Source: CAD feature listing. Evaluate the final solid. Frame: model axes, mm. Give positions to 0.01 mm unless a question says otherwise; leave off trailing zeros. Use one line per item in the form item = value. Start each with the question number.
(1) Cut plane A-A, the plane z = 1.5. Count the separate pieces of the cut face and the enclosed holes in it, and give its area (3 significant figures).
(2) Material intervals for line 1 along X through (y, z) = (-18, 1.85); line 2 along X through (y, z) = (-4.5, 5); line 3 along Y through (x, z) = (-198.5, 1.2), sorted ascending. Write a range as from..to.
(3) First-contact query: P1, Ø3, axis at x = 50.5, z = 3.5, coming from the +Y side; P2, Ø3, axis at x = 115, z = 0.5, coming from the -Y side; P3, Ø1.5, axis at y = -2.5, z = 3.5, coming from the -X side. Flat tips, straight axial feed; report the tip coordinate or a pass-through.
from build123d import *

# Parameters (mm, degrees)
SKETCH1_W           = 790
SKETCH1_H           = 80
BOSS_EXTRUDE1_DEPTH = 6
SKETCH2_W           = 25
SKETCH2_H           = 6
BOSS_EXTRUDE2_DEPTH = 6
SKETCH3_W           = 25
SKETCH3_H           = 6
SKETCH3_W_2         = 30
BOSS_EXTRUDE3_DEPTH = 6
CUT_EXTRUDE1_DEPTH  = 6
SKETCH5_W           = 6
SKETCH5_H           = 15
SKETCH5_H_2         = 20
CUT_EXTRUDE2_DEPTH  = 6
SKETCH7_W           = 6
SKETCH7_H           = 15
SKETCH7_H_2         = 20
CUT_EXTRUDE3_DEPTH  = 6
SKETCH8_W           = 30
SKETCH8_H           = 6
BOSS_EXTRUDE6_DEPTH = 6
SKETCH9_W           = 6
SKETCH9_H           = 20
SKETCH9_H_2         = 15
CUT_EXTRUDE4_DEPTH  = 6


with BuildPart() as part:
    # Sketch1 → Boss-Extrude1 (new body)
    with BuildSketch(Plane.XY):
        Rectangle(SKETCH1_W, SKETCH1_H)
    extrude(amount=BOSS_EXTRUDE1_DEPTH)

    # Sketch2 → Boss-Extrude2 (add)
    with BuildSketch(Plane(origin=(0, 40, 0), x_dir=(1, 0, 0), z_dir=(0, 1, 0))):
        with Locations((362.5, -3)):
            Rectangle(SKETCH2_W, SKETCH2_H)
        with Locations((304.5, -3)):
            Rectangle(SKETCH2_W, SKETCH2_H)
        with Locations((246.5, -3)):
            Rectangle(SKETCH2_W, SKETCH2_H)
        with Locations((188.5, -3)):
            Rectangle(SKETCH2_W, SKETCH2_H)
        with Locations((130.5, -3)):
            Rectangle(SKETCH2_W, SKETCH2_H)
        with Locations((72.5, -3)):
            Rectangle(SKETCH2_W, SKETCH2_H)
        with Locations((14.5, -3)):
            Rectangle(SKETCH2_W, SKETCH2_H)
        with Locations((-43.5, -3)):
            Rectangle(SKETCH2_W, SKETCH2_H)
        with Locations((-101.5, -3)):
            Rectangle(SKETCH2_W, SKETCH2_H)
        with Locations((-159.5, -3)):
            Rectangle(SKETCH2_W, SKETCH2_H)
        with Locations((-217.5, -3)):
            Rectangle(SKETCH2_W, SKETCH2_H)
        with Locations((-275.5, -3)):
            Rectangle(SKETCH2_W, SKETCH2_H)
    extrude(amount=BOSS_EXTRUDE2_DEPTH)

    # Sketch3 → Boss-Extrude3 (add)
    with BuildSketch(Plane.XZ.offset(40)):
        with Locations((-275.5, 3)):
            Rectangle(SKETCH3_W, SKETCH3_H)
        with Locations((-217.5, 3)):
            Rectangle(SKETCH3_W, SKETCH3_H)
        with Locations((-159.5, 3)):
            Rectangle(SKETCH3_W, SKETCH3_H)
        with Locations((-101.5, 3)):
            Rectangle(SKETCH3_W, SKETCH3_H)
        with Locations((-43.5, 3)):
            Rectangle(SKETCH3_W, SKETCH3_H)
        with Locations((14.5, 3)):
            Rectangle(SKETCH3_W, SKETCH3_H)
        with Locations((72.5, 3)):
            Rectangle(SKETCH3_W, SKETCH3_H)
        with Locations((130.5, 3)):
            Rectangle(SKETCH3_W, SKETCH3_H)
        with Locations((188.5, 3)):
            Rectangle(SKETCH3_W, SKETCH3_H)
        with Locations((246.5, 3)):
            Rectangle(SKETCH3_W, SKETCH3_H)
        with Locations((304.5, 3)):
            Rectangle(SKETCH3_W, SKETCH3_H)
        with Locations((362.5, 3)):
            Rectangle(SKETCH3_W, SKETCH3_H)
        with Locations((-350, 3)):
            Rectangle(SKETCH3_W_2, SKETCH3_H)
    extrude(amount=BOSS_EXTRUDE3_DEPTH)

    # Sketch4 → Cut-Extrude1 (cut)
    with BuildSketch(Plane(origin=(0, 0, 0), x_dir=(-1, 0, 0), z_dir=(0, 0, -1))):
        with BuildLine():
            Line((378, 17), (303, 17))
            ThreePointArc((303, 17), (299.464466094, 18.464466094), (298, 22))
            Line((298, 22), (298, 27))
            ThreePointArc((298, 27), (299.464466094, 30.535533906), (303, 32))
            Line((303, 32), (378, 32))
            ThreePointArc((378, 32), (381.535533906, 30.535533906), (383, 27))
            Line((383, 27), (383, 22))
            ThreePointArc((383, 22), (381.535533906, 18.464466094), (378, 17))
        make_face()
    extrude(amount=-CUT_EXTRUDE1_DEPTH, mode=Mode.SUBTRACT)

    # Sketch5 → Cut-Extrude2 (cut)
    with BuildSketch(Plane.ZY.offset(395)):
        with Locations((3, -32.5)):
            Rectangle(SKETCH5_W, SKETCH5_H)
        with Locations((3, 0)):
            Rectangle(SKETCH5_W, SKETCH5_H_2)
        with Locations((3, 32.5)):
            Rectangle(SKETCH5_W, SKETCH5_H)
    extrude(amount=-CUT_EXTRUDE2_DEPTH, mode=Mode.SUBTRACT)

    # Sketch7 → Cut-Extrude3 (cut)
    with BuildSketch(Plane(origin=(395, 0, 0), x_dir=(0, 0, -1), z_dir=(1, 0, 0))):
        with Locations((-3, 32.5)):
            Rectangle(SKETCH7_W, SKETCH7_H)
        with Locations((-3, 0)):
            Rectangle(SKETCH7_W, SKETCH7_H_2)
        with Locations((-3, -32.5)):
            Rectangle(SKETCH7_W, SKETCH7_H)
    extrude(amount=-CUT_EXTRUDE3_DEPTH, mode=Mode.SUBTRACT)

    # Sketch8 → Boss-Extrude6 (add)
    with BuildSketch(Plane(origin=(0, 40, 0), x_dir=(1, 0, 0), z_dir=(0, 1, 0))):
        with Locations((-350, -3)):
            Rectangle(SKETCH8_W, SKETCH8_H)
    extrude(amount=BOSS_EXTRUDE6_DEPTH)

    # Sketch9 → Cut-Extrude4 (cut)
    with BuildSketch(Plane.XY.offset(6)):
        with Locations((166, 0)):
            Rectangle(SKETCH9_W, SKETCH9_H)
        with Locations((282, 0)):
            Rectangle(SKETCH9_W, SKETCH9_H)
        with Locations((166, -22.5)):
            Rectangle(SKETCH9_W, SKETCH9_H_2)
        with Locations((166, 22.5)):
            Rectangle(SKETCH9_W, SKETCH9_H_2)
        with Locations((50, 0)):
            Rectangle(SKETCH9_W, SKETCH9_H)
        with Locations((50, -22.5)):
            Rectangle(SKETCH9_W, SKETCH9_H_2)
        with Locations((282, -22.5)):
            Rectangle(SKETCH9_W, SKETCH9_H_2)
        with Locations((282, 22.5)):
            Rectangle(SKETCH9_W, SKETCH9_H_2)
        with Locations((50, 22.5)):
            Rectangle(SKETCH9_W, SKETCH9_H_2)
        with Locations((-66, 0)):
            Rectangle(SKETCH9_W, SKETCH9_H)
        with Locations((-66, -22.5)):
            Rectangle(SKETCH9_W, SKETCH9_H_2)
        with Locations((-66, 22.5)):
            Rectangle(SKETCH9_W, SKETCH9_H_2)
        with Locations((-182, 0)):
            Rectangle(SKETCH9_W, SKETCH9_H)
        with Locations((-182, -22.5)):
            Rectangle(SKETCH9_W, SKETCH9_H_2)
        with Locations((-182, 22.5)):
            Rectangle(SKETCH9_W, SKETCH9_H_2)
    extrude(amount=-CUT_EXTRUDE4_DEPTH, mode=Mode.SUBTRACT)


solid = part.part
Geometry says:
q1.separate_pieces = 1
q1.enclosed_holes = 16
q1.area = 63,800 mm^2
q2.line_1 = -395..-185, -179..-69, -63..47, 53..163, 169..279, 285..395
q2.line_2 = -389..-185, -179..-69, -63..47, 53..163, 169..279, 285..389
q2.line_3 = -40..40
q3.P1 = 40
q3.P2 = -40
q3.P3 = -389
